```python
from build123d import *

# Parameters (mm, degrees)
F0_W      = 127
F0_H      = 127
F0_W_2    = 114.3
F0_H_2    = 114.3
F1_DEPTH  = 127
F2_W      = 25.4
F2_H      = 25.4
F3_DEPTH  = 6.35
F6_COUNT  = 4
F7_R      = 5.08
F9_DEPTH  = 7.62
F11_DEPTH = 127


with BuildPart() as f1:
    # F0 (on Top) → F1 (new body)
    with BuildSketch(Plane.XY):
        with Locations((-0.4615932703, 33.8642211668)):
            Rectangle(F0_W, F0_H)
        with Locations((-0.4615932703, 33.8642211668)):
            Rectangle(F0_W_2, F0_H_2, mode=Mode.SUBTRACT)
    extrude(amount=F1_DEPTH)

    # F2 (on face) → F3 (cut, through all)
    with BuildSketch(Plane.YZ.offset(63.0384067297)):
        with Locations((33.8642211668, 63.5)):
            Rectangle(F2_W, F2_H)
    f3 = extrude(amount=-F3_DEPTH, mode=Mode.SUBTRACT)

    # F6: F3 ×4 about axis
    f6_axis = Axis((-0.4615932703, 33.8642211668, 78.3742320016), (0, 0, -1))
    for i in range(1, F6_COUNT):
        add(f3.rotate(f6_axis, i * 360 / F6_COUNT), mode=Mode.SUBTRACT)

    # F7
    f7_edges = [f1.edges().sort_by_distance(p)[0] for p in [
        (-63.961593, -29.635779, 63.5),
        (63.038407, -29.635779, 63.5),
        (-63.961593, 97.364221, 63.5),
        (56.688407, 91.014221, 63.5),
        (63.038407, 97.364221, 63.5),
        (-57.611593, 91.014221, 63.5),
        (-57.611593, -23.285779, 63.5),
        (56.688407, -23.285779, 63.5),
    ]]
    fillet(f7_edges, radius=F7_R)

    # F8 (on face) → F9 (join)
    with BuildSketch(Plane.XY.offset(127)):
        with BuildLine():
            ThreePointArc((63.0384067297, -24.5557788332), (61.5505091781, -28.1478812816), (57.9584067297, -29.6357788332))
            Line((57.9584067297, -29.6357788332), (75.2250626683, -29.6357788332))
            Line((75.2250626683, -29.6357788332), (75.2250626683, 97.3642211668))
            Line((75.2250626683, 97.3642211668), (57.9584067297, 97.3642211668))
            ThreePointArc((57.9584067297, 97.3642211668), (61.5505091781, 95.8763236152), (63.0384067297, 92.2842211668))
            Line((63.0384067297, 92.2842211668), (63.0384067297, -24.5557788332))
        make_face()
        with BuildLine():
            ThreePointArc((-63.9615932703, -24.5557788332), (-62.4736957187, -28.1478812816), (-58.8815932703, -29.6357788332))
            Line((-58.8815932703, -29.6357788332), (57.9584067297, -29.6357788332))
            ThreePointArc((57.9584067297, -29.6357788332), (61.5505091781, -28.1478812816), (63.0384067297, -24.5557788332))
            Line((63.0384067297, -24.5557788332), (63.0384067297, 92.2842211668))
            ThreePointArc((63.0384067297, 92.2842211668), (61.5505091781, 95.8763236152), (57.9584067297, 97.3642211668))
            Line((57.9584067297, 97.3642211668), (-58.8815932703, 97.3642211668))
            ThreePointArc((-58.8815932703, 97.3642211668), (-62.4736957187, 95.8763236152), (-63.9615932703, 92.2842211668))
            Line((-63.9615932703, 92.2842211668), (-63.9615932703, -24.5557788332))
        make_face()
        with BuildLine():
            ThreePointArc((-52.5315932703, -23.2857788332), (-56.1236957187, -21.7978812816), (-57.6115932703, -18.2057788332))
            Line((-57.6115932703, -18.2057788332), (-57.6115932703, 85.9342211668))
            ThreePointArc((-57.6115932703, 85.9342211668), (-56.1236957187, 89.5263236152), (-52.5315932703, 91.0142211668))
            Line((-52.5315932703, 91.0142211668), (51.6084067297, 91.0142211668))
            ThreePointArc((51.6084067297, 91.0142211668), (55.2005091781, 89.5263236152), (56.6884067297, 85.9342211668))
            Line((56.6884067297, 85.9342211668), (56.6884067297, -18.2057788332))
            ThreePointArc((56.6884067297, -18.2057788332), (55.2005091781, -21.7978812816), (51.6084067297, -23.2857788332))
            Line((51.6084067297, -23.2857788332), (-52.5315932703, -23.2857788332))
        make_face(mode=Mode.SUBTRACT)
        with BuildLine():
            Line((-57.6115932703, 85.9342211668), (-57.6115932703, -18.2057788332))
            ThreePointArc((-57.6115932703, -18.2057788332), (-56.1236957187, -21.7978812816), (-52.5315932703, -23.2857788332))
            Line((-52.5315932703, -23.2857788332), (51.6084067297, -23.2857788332))
            ThreePointArc((51.6084067297, -23.2857788332), (55.2005091781, -21.7978812816), (56.6884067297, -18.2057788332))
            Line((56.6884067297, -18.2057788332), (56.6884067297, 85.9342211668))
            ThreePointArc((56.6884067297, 85.9342211668), (55.2005091781, 89.5263236152), (51.6084067297, 91.0142211668))
            Line((51.6084067297, 91.0142211668), (-52.5315932703, 91.0142211668))
            ThreePointArc((-52.5315932703, 91.0142211668), (-56.1236957187, 89.5263236152), (-57.6115932703, 85.9342211668))
        make_face()
        with BuildLine():
            Line((-74.7978676376, 97.3642211668), (-76.1525549474, -29.6357788332))
            Line((-76.1525549474, -29.6357788332), (-58.8815932703, -29.6357788332))
            ThreePointArc((-58.8815932703, -29.6357788332), (-62.4736957187, -28.1478812816), (-63.9615932703, -24.5557788332))
            Line((-63.9615932703, -24.5557788332), (-63.9615932703, 92.2842211668))
            ThreePointArc((-63.9615932703, 92.2842211668), (-62.4736957187, 95.8763236152), (-58.8815932703, 97.3642211668))
            Line((-58.8815932703, 97.3642211668), (-74.7978676376, 97.3642211668))
        make_face()
    extrude(amount=F9_DEPTH)

    # F10 (on face) → F11 (join, through all)
    with BuildSketch(Plane(origin=(0, 97.3642211668, 0), x_dir=(-1, 0, 0), z_dir=(0, 1, 0))):
        Polygon((0.1627568882, 235.1974227433), (-75.2250626683, 134.62), (74.3815182296, 134.62), align=None)
    extrude(amount=-F11_DEPTH)


solid = f1.part
```
Part model, mm, in its own coordinate system. A direction names the side the tool comes from. Round coordinates to 2 decimals unless told otherwise and drop trailing zeros. Order: outer loops, then holes, each group sorted by start corner. A loop starts at its lowest first (then second) coordinate and runs counter-clockwise, first axis right, second up. Notation, with made-up numbers: M 84.25,49 L 99.25,49 A11 cw 99.25,67 Z; hole C 3,77.25 d10. An arc over 180 degrees is marked long. Answer in a Markdown table with one row per item. Add a question column.
Q1. Cut at D-D on x = 22. Give the cut face in (y, z), and give its area (3 significant figures).
Q2. Cut at A-A on z = 104.5. Give the cut face in (x, y), and give its area (3 significant figures).
Q3. Pin check, flat tips, straight feed: pin 1 (3 mm diameter, centred on x = -60, z = 58.5, fed in from -Y); pin 2 (6 mm diameter, centred on x = -3.5, y = 33.5, fed in from -Z); pin 3 (1.9 mm diameter, centred on x = 60.5, y = 33.5, fed in from +Z); pin 4 (1.9 mm diameter, centred on x = -62, z = 61.5, fed in from +Y). Stop position of each tip, or through.
Q4. 3-axis set-ups, long thin cutter, end or side, ignore diameter. For faces 1 (the face through (-63.962, 20, 63)), 2 (the face through (60, 46.564, 63)), 3 (the face through (-56.08, 89.57, 64.39)), 4 (the face through (-1, -27, 50.8)): which of +Z, -Z, +X, -X, +Y, -Y reach the whole face in a straight line?
Q5. Wall check: L1, parallel to X at y = 73, z = 53; L2, parallel to Y at x = 23.5, z = 14; L3, parallel to Y at x = 53, z = 73. Give the ranges that are in metal, low to high. Write a range as from..to.
Q6. Cut at C-C on y = 37.5. Give the cut face in (x, z), and give its area (3 significant figures).
Q7. Cut at B-B on x = -5. Give the cut face in (y, z).
Q8. Mould opens along Z. For faces 5 (the face through (0, 94, 50.8)), 6 (the face through (56.688, 33, 48)), 7 (the face through (0, 94, 76.2)), 8 (the face through (70, 35, 127)) say: +Z half, -Z half, draft (parallel to the pull), parting line (faces both ways), or undercut.
Established:
| question | item | result |
|---|---|---|
| 1 | outline | M -29.64,0 L -23.29,0 L -23.29,127 L 91.01,127 L 91.01,0 L 97.36,0 L 97.36,205.63 L -29.64,205.63 Z |
| 1 | area | 11,600 mm2 |
| 2 | outline | M -63.96,-24.56 A5.08 ccw -58.88,-29.64 L 57.96,-29.64 A5.08 ccw 63.04,-24.56 L 63.04,92.28 A5.08 ccw 57.96,97.36 L -58.88,97.36 A5.08 ccw -63.96,92.28 Z; hole M -57.61,-18.21 A5.08 ccw -52.53,-23.29 L 51.61,-23.29 A5.08 ccw 56.69,-18.21 L 56.69,85.93 A5.08 ccw 51.61,91.01 L -52.53,91.01 A5.08 ccw -57.61,85.93 Z |
| 2 | area | 3,060 mm2 |
| 3 | pin 1 | stops at y = -29.64 |
| 3 | pin 2 | stops at z = 127 |
| 3 | pin 3 | stops at z = 155.53 |
| 3 | pin 4 | stops at y = 96.88 |
| 4 | face 1 | -Z, -X, +Y, -Y |
| 4 | face 2 | +X, -X |
| 4 | face 3 | -Z |
| 4 | face 4 | +Y, -Y |
| 5 | L1 | x = -63.96..-57.61, 56.69..63.04 |
| 5 | L2 | y = -29.64..-23.29, 91.01..97.36 |
| 5 | L3 | y = -29.64..-23.09, 90.82..97.36 |
| 6 | outline | M -75.44,127 L -63.96,127 L -63.96,76.2 L -57.61,76.2 L -57.61,127 L 56.69,127 L 56.69,76.2 L 63.04,76.2 L 63.04,127 L 75.23,127 L 75.23,134.62 L -0.16,235.2 L -74.38,134.62 L -75.44,134.62 Z; M -63.96,0 L -57.61,0 L -57.61,50.8 L -63.96,50.8 Z; M 56.69,0 L 63.04,0 L 63.04,50.8 L 56.69,50.8 Z |
| 6 | area | 9,960 mm2 |
| 7 | outline | M -29.64,0 L -23.29,0 L -23.29,50.8 L -29.64,50.8 Z; M -29.64,76.2 L -23.29,76.2 L -23.29,127 L 91.01,127 L 91.01,76.2 L 97.36,76.2 L 97.36,228.64 L -29.64,228.64 Z; M 91.01,0 L 97.36,0 L 97.36,50.8 L 91.01,50.8 Z |
| 8 | face 5 | undercut |
| 8 | face 6 | draft |
| 8 | face 7 | undercut |
| 8 | face 8 | -Z half |
